from build123d import *

# Parameters (mm, degrees)
F0_R     = 8.7
F1_DEPTH = 1.7


with BuildPart() as f1:
    # F0 (on Top) → F1 (new body)
    with BuildSketch(Plane.XY):
        Circle(F0_R)
        with BuildLine():
            Line((-4.178502, 5.237377), (-2.976663, 3.155732))
            ThreePointArc((-2.976663, 3.155732), (-4.338107, 0), (-2.976663, -3.155732))
            Line((-2.976663, -3.155732), (-4.178502, -5.237377))
            ThreePointArc((-4.178502, -5.237377), (-6.7, 0), (-4.178502, 5.237377))
        make_face(mode=Mode.SUBTRACT)
        with BuildLine():
            ThreePointArc((-1.244613, -4.155732), (2.169054, -3.756911), (4.221276, -1))
            Line((4.221276, -1), (6.624953, -1))
            ThreePointArc((6.624953, -1), (3.35, -5.80237), (-2.446451, -6.237377))
            Line((-2.446451, -6.237377), (-1.244613, -4.155732))
        make_face(mode=Mode.SUBTRACT)
        with BuildLine():
            Line((6.624953, 1), (4.221276, 1))
            ThreePointArc((4.221276, 1), (2.169054, 3.756911), (-1.244613, 4.155732))
            Line((-1.244613, 4.155732), (-2.446451, 6.237377))
            ThreePointArc((-2.446451, 6.237377), (3.35, 5.80237), (6.624953, 1))
        make_face(mode=Mode.SUBTRACT)
    extrude(amount=F1_DEPTH)


solid = f1.part
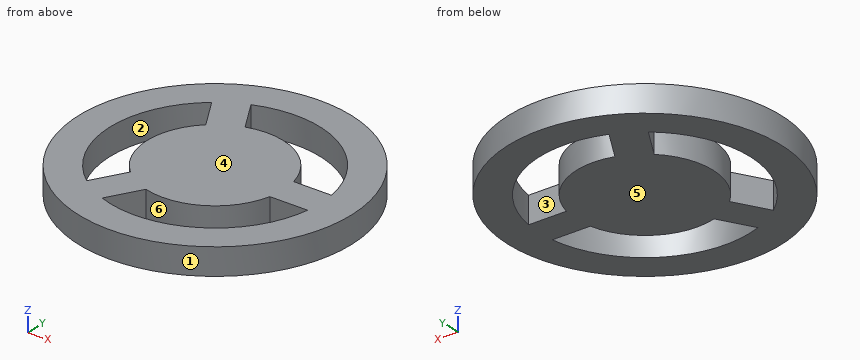
Input: part model. Units: mm. Frame: model coordinates. Face numbers are marked on the shaded views. A direction names the side the tool comes from. Give positions to 0.01 mm unless a question says otherwise; leave off trailing zeros. Write each loop counter-clockwise with the first axis right and the second up, starting at its lowest first coordinate (ties: lowest second). Pieces come first, ordered by that corner, then holes. Notation, with made-up numbers: M -2,18 L 26,18 A33 cw 26,52 Z; hole C 14.5,79.5 d5. An arc over 180 degrees is marked long. Write item = value, one per line. Start each with the question number.
1) Draft query along Y for the marked faces 1, 2, 3 and 4. Return one class per face: +Y half, -Y half, draft (parallel to the pull), parting line (faces both ways), or undercut.
2) Cut plane B-B on z = 1.3. Return the cut outline in (x, y), then the cut area to 3 significant figures.
3) Cut plane C-C on x = -2. Return the cut outline in (y, z), then the cut area to 3 significant figures.
4) Cut plane A-A on y = 0. Return the cut outline in (x, z).
5) Reachability of the marked faces 5 and 6 from +Z, -Z, +X, -X, +Y, -Y: full face, straight path, thin tool, end or side. Return the list, or none.
6) Cut plane D-D on x = -6. Return the cut outline in (y, z).
7) Material intervals for line 1 along Y through (x, z) = (0, 0.1); line 2 along Y through (x, z) = (2.75, 1.2); line 3 along X through (y, z) = (2.25, 0.1), sorted ascending. Write a range as [from, to].
Solved:
q1.face_1 = parting line
q1.face_2 = undercut
q1.face_3 = undercut
q1.face_4 = draft
q2.outline = C 0,0 d17.4; hole M -4.18,-5.24 L -2.98,-3.16 A4.34 cw -2.98,3.16 L -4.18,5.24 A6.7 ccw Z; hole M -2.45,-6.24 A6.7 ccw 6.62,-1 L 4.22,-1 A4.34 cw -1.24,-4.16 Z; hole M -2.45,6.24 L -1.24,4.16 A4.34 cw 4.22,1 L 6.62,1 A6.7 ccw Z
q2.area = 170 mm2
q3.outline = M -8.47,0 L -6.39,0 L -6.39,1.7 L -8.47,1.7 Z; M -5.46,0 L 5.46,0 L 5.46,1.7 L -5.46,1.7 Z; M 6.39,0 L 8.47,0 L 8.47,1.7 L 6.39,1.7 Z
q3.area = 25.6 mm2
q4.outline = M -8.7,0 L -6.7,0 L -6.7,1.7 L -8.7,1.7 Z; M -4.34,0 L 8.7,0 L 8.7,1.7 L -4.34,1.7 Z
q5.face_5 = -Z, +X, -X, +Y, -Y
q5.face_6 = +Z, -Z
q6.outline = M -6.3,0 L -2.98,0 L -2.98,1.7 L -6.3,1.7 Z; M 2.98,0 L 6.3,0 L 6.3,1.7 L 2.98,1.7 Z
q7.line_1 = [-8.7, -6.7], [-4.34, 4.34], [6.7, 8.7]
q7.line_2 = [-8.25, -6.11], [-3.36, 3.36], [6.11, 8.25]
q7.line_3 = [-8.4, -6.31], [-3.71, 3.71], [6.31, 8.4]
